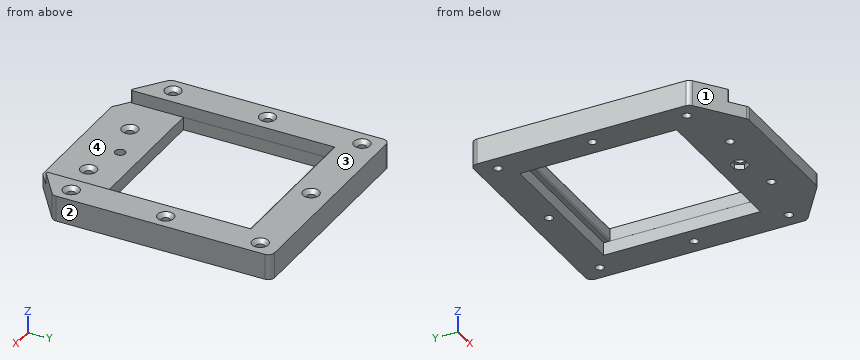
from build123d import *

# Parameters (mm, degrees)
BOSS_EXTRUDE1_DEPTH                                 = 10
BOSS_EXTRUDE2_DEPTH                                 = 10
FILLET1_R                                           = 1
FILLET2_R                                           = 4.999999999999999
FILLET3_R                                           = 1
SKETCH4_R                                           = 3.0000000000000018
SKETCH4_R_2                                         = 3.0000000000000027
SKETCH4_R_3                                         = 2.9999999999999862
SKETCH4_R_4                                         = 3.0000000000000266
SKETCH4_R_5                                         = 2.9999999999999947
SKETCH4_R_6                                         = 3.0000000000000044
SKETCH4_R_7                                         = 3.999999999999999
CUT_EXTRUDE1_DEPTH                                  = 20
CSK_FOR_M6_COUNTERSUNK_FLAT_HEAD_SCREW1_D           = 6.6
CSK_FOR_M6_COUNTERSUNK_FLAT_HEAD_SCREW1_CSINK_D     = 12.6
CSK_FOR_M6_COUNTERSUNK_FLAT_HEAD_SCREW1_CSINK_ANGLE = 90
CSK_FOR_M6_COUNTERSUNK_FLAT_HEAD_SCR_2_D            = 6.6
CSK_FOR_M6_COUNTERSUNK_FLAT_HEAD_SCR_2_CSINK_D      = 12.6
CSK_FOR_M6_COUNTERSUNK_FLAT_HEAD_SCR_2_CSINK_ANGLE  = 90
CUT_EXTRUDE2_DEPTH                                  = 4


with BuildPart() as part:
    # Sketch1 → Boss-Extrude1 (new body)
    with BuildSketch(Plane.XY):
        Polygon((-64.18159055149353, 136.6499257706783), (-64.18159055149351, -33.350074229321706), (-28.18019077559496, -60.35007422932169), (71.81700967260791, -60.35007422932168), (107.81840944850644, -33.350074229321706), (107.81840944850646, 136.64992577067832), align=None)
        Polygon((82.81840944850644, 111.64992577067832), (82.81840944850646, -10.350074229321688), (-39.18159055149353, -10.350074229321688), (-39.181590551493535, 111.64992577067831), align=None, mode=Mode.SUBTRACT)
    extrude(amount=BOSS_EXTRUDE1_DEPTH)

    # Sketch2 → Boss-Extrude2 (add)
    with BuildSketch(Plane.XY.offset(10)):
        Polygon((-64.18159055149353, 136.6499257706783), (107.81840944850646, 136.6499257706783), (107.8184094485065, -33.350074229321685), (82.81253069213544, -52.103754103569464), (82.81253069213545, 106.64992577067831), (-39.17571179512253, 106.64992577067831), (-39.17571179512251, -52.103754103569464), (-64.18159055149351, -33.350074229321706), align=None)
    extrude(amount=BOSS_EXTRUDE2_DEPTH)

    # Fillet1
    fillet1_edges = [part.edges().sort_by_distance(p)[0] for p in [
        (21.818409448506458, 106.64992577067831, 10),
        (21.818409448506458, 106.64992577067831, 20),
    ]]
    fillet(fillet1_edges, radius=FILLET1_R)

    # Fillet2
    fillet2_edges = [part.edges().sort_by_distance(p)[0] for p in [
        (-28.18019077559496, -60.35007422932169, 5),
        (-64.18159055149351, -33.350074229321706, 10),
        (-64.18159055149353, 136.6499257706783, 10),
        (71.81700967260791, -60.35007422932168, 5),
        (107.81840944850647, -33.35007422932169, 10),
        (107.81840944850646, 136.6499257706783, 10),
    ]]
    fillet(fillet2_edges, radius=FILLET2_R)

    # Fillet3
    fillet3_edges = [part.edges().sort_by_distance(p)[0] for p in [
        (82.81253069213544, -52.103754103569464, 15),
        (-39.17571179512251, -52.103754103569464, 15),
    ]]
    fillet(fillet3_edges, radius=FILLET3_R)

    # Sketch4 → Cut-Extrude1 (cut)
    with BuildSketch(Plane.XY.offset(20)):
        with Locations((-52.18159055149353, 121.64992577067831)):
            Circle(SKETCH4_R)
        with Locations((-52.18159055149302, -25.350074229321695)):
            Circle(SKETCH4_R)
        with Locations((-52.181590551493514, 48.14992577067831)):
            Circle(SKETCH4_R)
        with Locations((-8.181590551493347, -35.350074229321685)):
            Circle(SKETCH4_R_2)
        with Locations((51.81840944850665, -35.35007422932168)):
            Circle(SKETCH4_R_3)
        with Locations((95.81840944850728, 48.149925770678834)):
            Circle(SKETCH4_R_4)
        with Locations((95.81840944850728, -25.350074229321194)):
            Circle(SKETCH4_R_5)
        with Locations((95.81840944850677, 121.64992577067882)):
            Circle(SKETCH4_R_6)
        with Locations((21.818409448506646, -26.850074229321688)):
            Circle(SKETCH4_R_7)
        with Locations((21.818409448506618, 121.64992577067856)):
            Circle(SKETCH4_R)
    extrude(amount=-CUT_EXTRUDE1_DEPTH, mode=Mode.SUBTRACT)

    # CSK for M6 Countersunk Flat Head Screw1 (through all)
    with Locations(Plane(origin=(-52.181590551, 121.649925771, 20), x_dir=(1, 0, 0), z_dir=(0, 0, 1))):
        with Locations((0, 0), (0, -73.5), (0, -147), (148, -147), (148, -73.5), (148, 0), (74, 0)):
            CounterSinkHole(CSK_FOR_M6_COUNTERSUNK_FLAT_HEAD_SCREW1_D / 2, CSK_FOR_M6_COUNTERSUNK_FLAT_HEAD_SCREW1_CSINK_D / 2, counter_sink_angle=CSK_FOR_M6_COUNTERSUNK_FLAT_HEAD_SCREW1_CSINK_ANGLE)

    # CSK for M6 Countersunk Flat Head Scr 2 (through all)
    with Locations(Plane(origin=(-8.181590551, -35.350074229, 10), x_dir=(1, 0, 0), z_dir=(0, 0, 1))):
        with Locations((0, 0), (60, 0)):
            CounterSinkHole(CSK_FOR_M6_COUNTERSUNK_FLAT_HEAD_SCR_2_D / 2, CSK_FOR_M6_COUNTERSUNK_FLAT_HEAD_SCR_2_CSINK_D / 2, counter_sink_angle=CSK_FOR_M6_COUNTERSUNK_FLAT_HEAD_SCR_2_CSINK_ANGLE)

    # Sketch6 → Cut-Extrude2 (cut)
    with BuildSketch(Plane(origin=(0, 0, 0), x_dir=(-1, 0, 0), z_dir=(0, 0, -1))):
        Polygon((-14.890206218231118, -26.850074229321667), (-18.354307833368882, -20.850074229321656), (-25.282511063644392, -20.850074229321656), (-28.74661267878215, -26.850074229321656), (-25.282511063644392, -32.850074229321656), (-18.354307833368868, -32.850074229321656), align=None)
    extrude(amount=-CUT_EXTRUDE2_DEPTH, mode=Mode.SUBTRACT)


solid = part.part
The listing builds one solid part. Answer for the finished solid, in the listing's coordinates (mm). Face numbers are marked on the shaded views. Round coordinates to 2 decimals unless told otherwise and drop trailing zeros. Order: outer loops, then holes, each group sorted by start corner. A loop starts at its lowest first (then second) coordinate and runs counter-clockwise, first axis right, second up. Notation, with made-up numbers: (62, 2.5) -> (90, 2.5) arc R13 cw to (90, 27.5) -> close; hole circle Ø10 at (-17.5, 75.25). An arc over 180 degrees is marked (long way). One line per item, written item: value.
Item 1: Find section C-C, the plane x = 21. State how many separate pieces and enclosed holes the cut face has, then the cut area to 3 significant figures.
Taken from the geometry:
separate pieces: 4
enclosed holes: 0
area: 818 mm2
Item 2: For a pull along X with two mould halves and no side action, classify the marked faces 1, 2, 3 and 4 as released by +X, released by -X, zero draft, split by the parting line, or undercut.
Taken from the geometry:
face 1: released by -X
face 2: released by +X
face 3: zero draft
face 4: undercut
Item 3: Straight lines are drawn through the part: L1, parallel to X at y = 49.5, z = 17.25; L2, parallel to X at y = -1, z = 5.75; L3, parallel to X at y = 46.5, z = 16.5. For each, find the intervals that lie inside material, in ascending order.
Taken from the geometry:
L1: x = -64.18 to -55.46, -48.9 to -39.18, 82.81 to 92.54, 99.1 to 107.82
L2: x = -64.18 to -39.18, 82.82 to 107.82
L3: x = -64.18 to -55.04, -49.32 to -39.18, 82.81 to 92.96, 98.68 to 107.82
Item 4: Given P1, Ø10, axis at y = -39.5, z = 13.5, coming from the +X side; P2, Ø8.5, axis at x = -52.18, y = 121.65, coming from the +Z side; P3, Ø6.5, axis at x = 27.5, z = 14, coming from the -Y side, each flat-ended and moving along its own axis, determine where each tip first touches the part or whether it passes through.
Taken from the geometry:
P1: stops at x = 106.24
P2: stops at z = 17.95
P3: stops at y = 106.65
Item 5: Find section B-B, the plane x = 39. Give the vertices of the cut face in (y, z).
Taken from the geometry:
outline: (-60.35, 0) -> (-10.35, 0) -> (-10.35, 10) -> (-60.35, 10) -> close; (106.65, 11) arc R1 ccw to (107.65, 10) -> (111.65, 10) -> (111.65, 0) -> (136.65, 0) -> (136.65, 20) -> (107.65, 20) arc R1 ccw to (106.65, 19) -> close
